The model under review builds one solid part; all positions refer to its coordinate system, in mm. Round coordinates to 2 decimals unless told otherwise and drop trailing zeros. Write each loop counter-clockwise with the first axis right and the second up, starting at its lowest first coordinate (ties: lowest second). Pieces come first, ordered by that corner, then holes. Notation, with made-up numbers: (-16, -26.5) - (7, -26.5) arc R20 cw to (7, 3.5) - close; hole circle Ø5 at (38, 20). An arc over 180 degrees is marked (long way). Return JSON: item names as keys, results as strings.
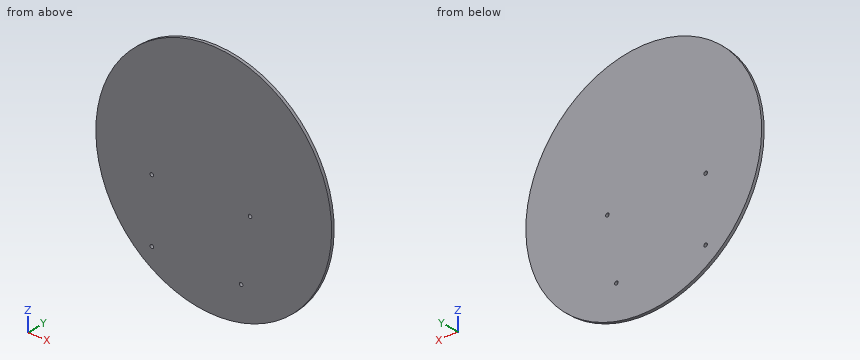
from build123d import *

# Parameters (mm, degrees)
SKETCH1_R           = 99
BOSS_EXTRUDE1_DEPTH = 2.5
SKETCH2_R           = 96.5
CUT_EXTRUDE1_DEPTH  = 2.5
SKETCH3_R           = 96.5
SKETCH3_R_2         = 1.5
BOSS_EXTRUDE3_DEPTH = 2.5


with BuildPart() as part:
    # Sketch1 → Boss-Extrude1 (new body)
    with BuildSketch(Plane(origin=(0, 0, 0), x_dir=(1, 0, 0), z_dir=(0, 1, 0))):
        with Locations(Location((0, 0, 0), (0, 0, 270))):
            Circle(SKETCH1_R)
    extrude(amount=BOSS_EXTRUDE1_DEPTH)

    # Sketch2 → Cut-Extrude1 (cut)
    with BuildSketch(Plane(origin=(0, 2.5, 0), x_dir=(1, 0, 0), z_dir=(0, 1, 0))):
        with Locations(Location((0, 0, 0), (0, 0, 270))):
            Circle(SKETCH2_R)
    extrude(amount=-CUT_EXTRUDE1_DEPTH, mode=Mode.SUBTRACT)

    # Sketch3 → Boss-Extrude3 (add)
    with BuildSketch(Plane(origin=(0, 2.5, 0), x_dir=(1, 0, 0), z_dir=(0, 1, 0))):
        Circle(SKETCH3_R)
        with Locations(Location((-52.01148814, 14.941708329, 0), (0, 0, 270))):
            Circle(SKETCH3_R_2, mode=Mode.SUBTRACT)
        with Locations(Location((-52.01148814, 67.941708329, 0), (0, 0, 270))):
            Circle(SKETCH3_R_2, mode=Mode.SUBTRACT)
        with Locations(Location((22.98851186, 67.941708329, 0), (0, 0, 270))):
            Circle(SKETCH3_R_2, mode=Mode.SUBTRACT)
        with Locations(Location((30.48851186, 14.941708329, 0), (0, 0, 270))):
            Circle(SKETCH3_R_2, mode=Mode.SUBTRACT)
    extrude(amount=-BOSS_EXTRUDE3_DEPTH)


solid = part.part
(1) Clearance check with flat-ended pins moving along their axes: pin 1 Ø1.8 at (x, z) = (22.99, -67.94) entering from -Y; pin 2 Ø1.5 at (y, z) = (1.5, 55) entering from -X. State where each tip first meets the part, or that it passes through.
Filled in:
{"pin 1": "passes through", "pin 2": "stops at x = -82.81"}
(2) Add section B-B (x = 51.5). Write out the cut boundary in (y, z), plus the area to 3 significant figures.
Filled in:
{"outline": "(0, -84.55) - (2.5, -84.55) - (2.5, 84.55) - (0, 84.55) - close", "area": "423 mm2"}
(3) Wall thickness on line 1 (X direction, y = 0.7, z = -68); line 2 (X direction, y = 1.3, z = -70); line 3 (Z direction, x = 61.5, y = 1.5): over which ranges is each line inside the solid? List them lowest first.
Filled in:
{"line 1": "x = -71.95 to -53.51, -50.51 to 21.49, 24.49 to 71.95", "line 2": "x = -70.01 to 70.01", "line 3": "z = -77.58 to 77.58"}
(4) Add section A-A (y = 1.2). Write out the cut boundary in (x, z), plus the area to 3 significant figures.
Filled in:
{"outline": "circle Ø198 at (0, 0); hole circle Ø3 at (-52.01, -67.94); hole circle Ø3 at (-52.01, -14.94); hole circle Ø3 at (22.99, -67.94); hole circle Ø3 at (30.49, -14.94)", "area": "30,800 mm2"}
(5) Add section C-C (z = 85.5). Write out the cut boundary in (x, y).
Filled in:
{"outline": "(-49.91, 0) - (49.91, 0) - (49.91, 2.5) - (-49.91, 2.5) - close"}
